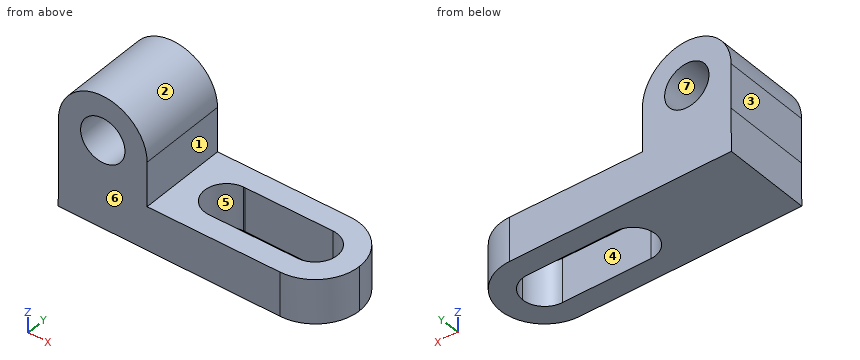
from build123d import *

# Parameters (mm, degrees)
F1_DEPTH = 25.4
F2_R     = 6.3498502592
F3_DEPTH = 25.4
F5_DEPTH = 12.7
F7_DEPTH = 25.4


with BuildPart() as f1:
    # F0 (on Front) → F1 (new body)
    with BuildSketch(Plane.XZ):
        with BuildLine():
            Line((-29.9805339301, 47.0739776071), (-29.9805339301, 34.3739776071))
            Line((-29.9805339301, 34.3739776071), (-30.0404094228, 22.0440076031))
            Line((-30.0404094228, 22.0440076031), (46.1586921323, 21.6739776071))
            Line((46.1586921323, 21.6739776071), (46.1586921323, 34.3739776071))
            Line((46.1586921323, 34.3739776071), (-4.5808334117, 34.3739776071))
            Line((-4.5808334117, 34.3739776071), (-4.5808334117, 47.0739776071))
            ThreePointArc((-4.5808334117, 47.0739776071), (-17.2806836709, 59.7738278663), (-29.9805339301, 47.0739776071))
        make_face()
    extrude(amount=F1_DEPTH)

    # F2 (on face) → F3 (cut)
    with BuildSketch(Plane.XZ.offset(25.4)):
        with Locations((-17.2806836709, 47.0739776071)):
            Circle(F2_R)
    extrude(amount=-F3_DEPTH, mode=Mode.SUBTRACT)

    # F4 (on face) → F5 (cut)
    with BuildSketch(Plane.XY.offset(34.3739776071)):
        with BuildLine():
            ThreePointArc((33.4586921323, 0), (42.4389482533, -3.7197438789), (46.1586921323, -12.7))
            Line((46.1586921323, -12.7), (46.1586921323, 0))
            Line((46.1586921323, 0), (33.4586921323, 0))
        make_face()
        with BuildLine():
            Line((46.1586921323, -25.4), (46.1586921323, -12.7))
            ThreePointArc((46.1586921323, -12.7), (42.4389482533, -21.6802561211), (33.4586921323, -25.4))
            Line((33.4586921323, -25.4), (46.1586921323, -25.4))
        make_face()
    extrude(amount=-F5_DEPTH, mode=Mode.SUBTRACT)

    # F6 (on face) → F7 (cut)
    with BuildSketch(Plane.XY.offset(34.3739776071)):
        with BuildLine():
            Line((8.3943191118, -6.3559641324), (7.8409948456, -6.3560958014))
            ThreePointArc((7.8409948456, -6.3560958014), (1.7706907215, -12.8391192629), (8.1191665883, -19.05))
            ThreePointArc((8.1191665883, -19.05), (12.6092946488, -17.1901280605), (14.4691665883, -12.7))
            ThreePointArc((14.4691665883, -12.7), (12.7055441634, -8.308230341), (8.3943191118, -6.3559641324))
        make_face()
        with BuildLine():
            ThreePointArc((14.4691665883, -12.7), (12.6092946488, -17.1901280605), (8.1191665883, -19.05))
            Line((8.1191665883, -19.05), (33.4586921323, -19.05))
            ThreePointArc((33.4586921323, -19.05), (27.1086921772, -12.7007555222), (33.4571810878, -6.3500001798))
            Line((33.4571810878, -6.3500001798), (8.3943191118, -6.3559641324))
            ThreePointArc((8.3943191118, -6.3559641324), (12.7055441634, -8.308230341), (14.4691665883, -12.7))
        make_face()
        with BuildLine():
            ThreePointArc((33.4571810878, -6.3500001798), (27.1086921772, -12.7007555222), (33.4586921323, -19.05))
            ThreePointArc((33.4586921323, -19.05), (37.9488201928, -17.1901280605), (39.8086921323, -12.7))
            ThreePointArc((39.8086921323, -12.7), (37.9482859261, -8.2093377364), (33.4571810878, -6.3500001798))
        make_face()
    extrude(amount=-F7_DEPTH, mode=Mode.SUBTRACT)


solid = f1.part
Verification items for the finished model (mm, model axes). Face numbers are marked on the shaded views. A direction names the side the tool comes from. Give positions to 0.01 mm unless a question says otherwise; leave off trailing zeros. Loops run counter-clockwise (first coordinate to the right, second up) from the corner with the lowest first, then second, coordinate; pieces in that order, holes last.
1) Draft check along Y on the marked faces 4, 5, 6 and 7. Enter one of: pulls with the +Y half, pulls with the -Y half, needs draft (parallel to the pull), parting line crosses it, or undercut.
2) Sectioned sample at A-A, the plane y = -16.75. Enter the section's corners in (x, z).
3) Sectioned sample at C-C, the plane z = 44. Enter the section's corners in (x, y), then the cut area to 3 significant figures.
4) Thickness scan on line 1 along Y through (x, z) = (12, 34); line 2 along X through (y, z) = (-19.25, 39.5); line 3 along X through (y, z) = (-13, 30). Record the ranges inside material, lowest first.
5) Sectioned sample at B-B, the plane z = 51.5. Enter the section's corners in (x, y), then the cut area to 3 significant figures.
6) Depth check by flat-ended pin: pin 1 Ø5 at (y, z) = (-19.5, 42) entering from +X; pin 2 Ø5 at (x, z) = (36, 32.5) entering from -Y; pin 3 Ø1.5 at (y, z) = (-3, 31.5) entering from -X; pin 4 Ø2 at (y, z) = (-20, 51.5) entering from -X. Enter the tip coordinate at first touch or a pass-through.
7) Sectioned sample at D-D, the plane y = -20.25. Enter the section's corners in (x, z), then the cut area to 3 significant figures.
8) Set-up check for the marked faces 1, 2 and 3: record each of +Z, -Z, +X, -X, +Y, -Y from which the full face is reachable in a straight line by a thin tool's end or side.
Answers:
1. face 4: undercut
1. face 5: undercut
1. face 6: pulls with the -Y half
1. face 7: needs draft
2. outline: (-30.04, 22.04) - (3.23, 21.88) - (3.23, 34.37) - (-4.58, 34.37) - (-4.58, 47.07) arc R12.7 ccw to (-29.98, 47.07) - (-29.98, 34.37) - close; (38.35, 21.71) - (45.5, 21.68) - (45.5, 34.37) - (38.35, 34.37) - close; hole circle Ø12.7 at (-17.28, 47.07)
3. outline: (-29.98, -25.4) - (-22.84, -25.4) - (-22.84, 0) - (-29.98, 0) - close; (-11.72, -25.4) - (-4.58, -25.4) - (-4.58, 0) - (-11.72, 0) - close
3. area: 363 mm2
4. line 1: y = -25.4 to -19.05, -6.36 to 0
4. line 2: x = -29.98 to -4.58
4. line 3: x = -30 to 1.78, 39.8 to 46.16
5. outline: (-29.18, -25.4) - (-21.83, -25.4) - (-21.83, 0) - (-29.18, 0) - close; (-12.73, -25.4) - (-5.38, -25.4) - (-5.38, 0) - (-12.73, 0) - close
5. area: 373 mm2
6. pin 1: stops at x = -4.58
6. pin 2: stops at y = -25.4
6. pin 3: stops at x = -30
6. pin 4: stops at x = -29.51
7. outline: (-30.04, 22.04) - (43.67, 21.69) - (43.67, 34.37) - (-4.58, 34.37) - (-4.58, 47.07) arc R12.7 ccw to (-29.98, 47.07) - (-29.98, 34.37) - close; hole circle Ø12.7 at (-17.28, 47.07)
7. area: 1,370 mm2
8. face 1: +Z, +X, +Y, -Y
8. face 2: +Z, +Y, -Y
8. face 3: +Z, -X, +Y, -Y
